from build123d import *

# Parameters (mm, degrees)
SKETCH1_R           = 8
SKETCH1_R_2         = 2.5
BOSS_EXTRUDE1_DEPTH = 16
SKETCH2_W           = 2
SKETCH2_H           = 7
SKETCH3_R           = 1.55
CUT_EXTRUDE1_DEPTH  = 8
CIRPATTERN1_COUNT   = 2
CIRPATTERN1_ANGLE   = 90


with BuildPart() as part:
    # Sketch1 → Boss-Extrude1 (new body)
    with BuildSketch(Plane(origin=(0, 0, 0), x_dir=(1, 0, 0), z_dir=(0, 1, 0))):
        with Locations(Location((0, 0, 0), (0, 0, 270))):
            Circle(SKETCH1_R)
        with Locations(Location((0, 0, 0), (0, 0, 270))):
            Circle(SKETCH1_R_2, mode=Mode.SUBTRACT)
    extrude(amount=BOSS_EXTRUDE1_DEPTH)

    # Sketch2 → Cut-Revolve1 (revolve, cut)
    with BuildSketch(Plane.XY, mode=Mode.PRIVATE) as cut_revolve1_sk:
        with Locations((-7, 11.2)):
            Rectangle(SKETCH2_W, SKETCH2_H)
    revolve(cut_revolve1_sk.sketch.rotate(Axis((0, 16.938378215, 0), (0, -1, 0)), 270), axis=Axis((0, 16.938378215, 0), (0, -1, 0)), mode=Mode.SUBTRACT)

    # Sketch3 → Cut-Extrude1 (cut)
    with BuildSketch(Plane.ZY.offset(8)):
        with Locations((0, 3.7)):
            Circle(SKETCH3_R)
    cut_extrude1 = extrude(amount=-CUT_EXTRUDE1_DEPTH, mode=Mode.SUBTRACT)

    # CirPattern1: Cut-Extrude1 ×2 about axis
    cirpattern1_axis = Axis((0, 16, 0), (0, -1, 0))
    for i in range(1, CIRPATTERN1_COUNT):
        add(cut_extrude1.rotate(cirpattern1_axis, i * CIRPATTERN1_ANGLE / (CIRPATTERN1_COUNT - 1)), mode=Mode.SUBTRACT)


solid = part.part
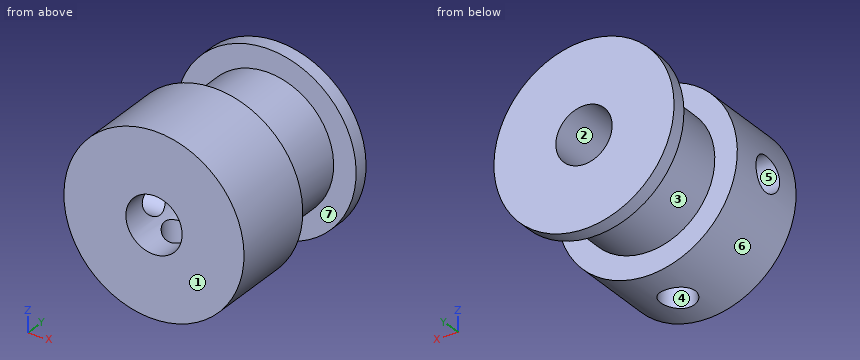
Geometry check sheet. Reference: the model listing, model coordinates, mm. Face numbers are marked on the shaded views. A direction names the side the tool comes from. Give positions to 0.01 mm unless a question says otherwise; leave off trailing zeros. Write each loop counter-clockwise with the first axis right and the second up, starting at its lowest first coordinate (ties: lowest second). Pieces come first, ordered by that corner, then holes. Notation, with made-up numbers: M 41,72.25 L 63,72.25 A33 cw 63,110.25 Z; hole C 57.25,28 d4. An arc over 180 degrees is marked long. One line per question, with ' | ' between items.
1. Cross-section at B-B (y = 3.7). Enter the section's corners in (x, z), plus the area to 3 significant figures.
Ans:
outline: M -7.85,-1.55 A8 ccw -1.55,-7.85 L -1.55,-1.96 A2.5 cw -1.96,-1.55 Z; M -7.85,1.55 L -1.96,1.55 A2.5 cw long 1.55,-1.96 L 1.55,-7.85 A8 ccw long Z | area: 147 mm2
2. Cross-section at C-C (x = 7). Enter the section's corners in (y, z).
Ans:
outline: M 0,-3.87 L 7.7,-3.87 L 7.7,3.87 L 0,3.87 Z; M 14.7,-3.87 L 16,-3.87 L 16,3.87 L 14.7,3.87 Z
3. Mould release check, pull along X, two halves, no side actions. Record for the marked faces 1, 2, 3 and 4: released by +X, released by -X, zero draft, split by the parting line, or undercut.
Ans:
face 1: zero draft | face 2: undercut | face 3: split by the parting line | face 4: undercut
4. Scan lines: line 1 along Y through (x, z) = (-4.25, -6.5); line 2 along X through (y, z) = (7.25, 0); line 3 along X through (y, z) = (7.75, 0). Record each from-to range of solid material in increasing order. Write a range as from..to.
Ans:
line 1: 0..7.7, 14.7..16 | line 2: -8..-2.5, 2.5..8 | line 3: -6..-2.5, 2.5..6
5. Gauge pin test, flat ends, axial feed: pin 1 (5 mm diameter, centred on y = 3.7, z = 0, fed in from -X); pin 2 (1.5 mm diameter, centred on y = 3.5, z = 5.5, fed in from +X); pin 3 (1.5 mm diameter, centred on y = 4, z = 4, fed in from -X); pin 4 (1 mm diameter, centred on x = 0.5, y = 14, fed in from +Z). Record the tip position at first contact, or that the pin passes through.
Ans:
pin 1: x = -8 | pin 2: x = 6.44 | pin 3: x = -7.31 | pin 4: z = 6
6. Cross-section at A-A (z = 0). Enter the section's corners in (x, y).
Ans:
outline: M -8,0 L -2.5,0 L -2.5,2.15 L -8,2.15 Z; M -8,5.25 L -2.5,5.25 L -2.5,16 L -8,16 L -8,14.7 L -6,14.7 L -6,7.7 L -8,7.7 Z; M 2.5,0 L 8,0 L 8,7.7 L 6,7.7 L 6,14.7 L 8,14.7 L 8,16 L 2.5,16 Z
7. Set-up check for the marked faces 5, 6 and 7: record each of +Z, -Z, +X, -X, +Y, -Y from which the full face is reachable in a straight line by a thin tool's end or side.
Ans:
face 5: -X | face 6: +Y, -Y | face 7: none
8. Cross-section at D-D (z = -5.5). Enter the section's corners in (x, y), plus the area to 3 significant figures.
Ans:
outline: M -5.81,0 L 5.81,0 L 5.81,7.7 L 2.4,7.7 L 2.4,14.7 L 5.81,14.7 L 5.81,16 L -5.81,16 L -5.81,14.7 L -2.4,14.7 L -2.4,7.7 L -5.81,7.7 Z; hole C 0,3.7 d3.1 | area: 131 mm2
